Build history of the part. All positions in model axes, mm. Round coordinates to 2 decimals unless told otherwise and drop trailing zeros. Write each loop counter-clockwise with the first axis right and the second up, starting at its lowest first coordinate (ties: lowest second). Pieces come first, ordered by that corner, then holes.
1) Saw through at B-B (z = 101.6). Write the cut outline in (x, y) (3 decimals).
2) Flat gauge pins, fed straight in: pin 1 (6 mm diameter, centred on x = 28.02, z = 190.5, fed in from -Y); pin 2 (1 mm diameter, centred on x = 18, y = 14.5, fed in from -Z). Where does each tip first touch, or does it go through?
3) Wall check: probe 1 along X at (y, z) = (14.9, 97.5); probe 2 along X at (y, z) = (14.85, 190.5); probe 3 along X at (y, z) = (13.85, 180). Give the ranges that are in metal, low to high.
4) Pull direction Z, two halves, no side cores. Call faces 1 (the flat face through (39.48, 14.27, 54.83)), 2 (the flat face through (-1, 12.7, 114)), 3 (the cylindrical face through (-54.223, 14.31, 115.586)), 4 (the cylindrical face through (28.89, 14.31, 192.19)): +Z half, -Z half, draft (parallel to the pull), parting line (faces both ways), or undercut.
5) Saw through at C-C (y = 15.15). State how many separate pieces and enclosed holes the cut face has, plus the area to 3 significant figures.
6) Saw through at A-A (x = -24.5). Write the cut outline in (y, z) (3 decimals).
7) Saw through at D-D (z = -4). Write the cut outline in (x, y) (3 decimals), plus the area to 3 significant figures.
from build123d import *

# Parameters (mm, degrees)
SKETCH3_W                = 114.3
SKETCH3_H                = 88.9
SKETCH3_W_2              = 101.6
SKETCH3_H_2              = 76.2
BOSS_EXTRUDE1_DEPTH      = 12.7
BOSS_EXTRUDE1_DEPTH_BACK = 12.7
SKETCH4_W                = 114.3
SKETCH4_H                = 88.9
BOSS_EXTRUDE2_DEPTH      = 3.175
BOSS_EXTRUDE3_DEPTH      = 3.175
SKETCH7_W                = 44.45
SKETCH7_H                = 25.4
BOSS_EXTRUDE4_DEPTH      = 6.35
SKETCH6_R                = 9.9695
CUT_EXTRUDE1_DEPTH       = 115.3
SKETCH13_W               = 29.21
SKETCH13_H               = 25.4
BOSS_EXTRUDE5_DEPTH      = 4.064
SKETCH14_W               = 6.35
SKETCH14_H               = 2.54
CUT_EXTRUDE2_DEPTH       = 31.75
SKETCH18_W               = 10.16
SKETCH18_H               = 5.08
CUT_EXTRUDE3_DEPTH       = 6.35
SKETCH19_R               = 0.635
CUT_EXTRUDE4_DEPTH       = 25.4
SKETCH20_R               = 1.905
CUT_EXTRUDE7_DEPTH       = 3.175
SKETCH23_R               = 5.08
SKETCH23_R_2             = 1.905
SKETCH23_R_3             = 2.38125
CUT_EXTRUDE8_DEPTH       = 3.175
SKETCH24_R               = 1.25
CUT_EXTRUDE9_DEPTH       = 3.175
BOSS_EXTRUDE7_DEPTH      = 114.3
BOSS_EXTRUDE8_DEPTH      = 28.575
SKETCH25_R               = 15.875
SKETCH25_R_2             = 12.7
CUT_EXTRUDE10_DEPTH      = 32.75
FILLET1_R                = 9.525
FILLET2_R                = 5.08
FILLET3_R                = 9.525


with BuildPart() as part:
    # Sketch3 → Boss-Extrude1 (new body, two sides)
    with BuildSketch(Plane(origin=(0, 0, 0), x_dir=(1, 0, 0), z_dir=(0, 1, 0))) as boss_extrude1_sk:
        with Locations((0, -158.75)):
            Rectangle(SKETCH3_W, SKETCH3_H)
        with Locations((0, -158.75)):
            Rectangle(SKETCH3_W_2, SKETCH3_H_2, mode=Mode.SUBTRACT)
    extrude(amount=BOSS_EXTRUDE1_DEPTH)
    extrude(boss_extrude1_sk.sketch, amount=-BOSS_EXTRUDE1_DEPTH_BACK)

    # Sketch4 → Boss-Extrude2 (add)
    with BuildSketch(Plane.XZ.offset(12.7)):
        with Locations((0, 158.75)):
            Rectangle(SKETCH4_W, SKETCH4_H)
    extrude(amount=BOSS_EXTRUDE2_DEPTH)

    # Sketch7 → Boss-Extrude4 (add)
    with BuildSketch(Plane(origin=(0, -12.7, 0), x_dir=(1, 0, 0), z_dir=(0, 1, 0))):
        with Locations((-28.575, -133.35)):
            Rectangle(SKETCH7_W, SKETCH7_H)
        with Locations((28.575, -133.35)):
            Rectangle(SKETCH7_W, SKETCH7_H)
    extrude(amount=BOSS_EXTRUDE4_DEPTH)

    # Sketch6 → Cut-Extrude1 (cut, through all)
    with BuildSketch(Plane.ZY.offset(57.15)):
        with Locations((133.35, 0)):
            Circle(SKETCH6_R)
    extrude(amount=-CUT_EXTRUDE1_DEPTH, mode=Mode.SUBTRACT)

    # Sketch13 → Boss-Extrude5 (add)
    with BuildSketch(Plane(origin=(0, -12.7, 0), x_dir=(1, 0, 0), z_dir=(0, 1, 0))):
        with Locations((-20.955, -133.35)):
            Rectangle(SKETCH13_W, SKETCH13_H)
        with Locations((20.955, -133.35)):
            Rectangle(SKETCH13_W, SKETCH13_H)
    extrude(amount=BOSS_EXTRUDE5_DEPTH)

    # Sketch14 → Cut-Extrude2 (cut)
    with BuildSketch(Plane.XY.offset(146.05)):
        with Locations((-27.305, -10.414)):
            Rectangle(SKETCH14_W, SKETCH14_H)
        with Locations((-27.305, -3.81)):
            Rectangle(SKETCH14_W, SKETCH14_H)
        with Locations((27.305, -10.414)):
            Rectangle(SKETCH14_W, SKETCH14_H)
        with Locations((27.305, -3.81)):
            Rectangle(SKETCH14_W, SKETCH14_H)
    extrude(amount=-CUT_EXTRUDE2_DEPTH, mode=Mode.SUBTRACT)

    # Sketch18 → Cut-Extrude3 (cut)
    with BuildSketch(Plane.XY.offset(120.65)):
        with Locations((-43.18, 10.16)):
            Rectangle(SKETCH18_W, SKETCH18_H)
    extrude(amount=-CUT_EXTRUDE3_DEPTH, mode=Mode.SUBTRACT)

    # Sketch19 → Cut-Extrude4 (cut)
    with BuildSketch(Plane(origin=(0, 12.7, 0), x_dir=(1, 0, 0), z_dir=(0, 1, 0))):
        with Locations((-53.975, -117.475)):
            Circle(SKETCH19_R)
        with Locations((53.975, -117.475)):
            Circle(SKETCH19_R)
        with Locations((-53.975, -200.025)):
            Circle(SKETCH19_R)
        with Locations((53.975, -200.025)):
            Circle(SKETCH19_R)
    extrude(amount=-CUT_EXTRUDE4_DEPTH, mode=Mode.SUBTRACT)

    # Sketch26 → Boss-Extrude7 (add)
    with BuildSketch(Plane(origin=(57.15, 0, 0), x_dir=(0, 0, -1), z_dir=(1, 0, 0))):
        Polygon((-203.2, 12.7), (-203.454, 12.7), (-203.454, 15.875), (-204.724, 15.875), (-213.23138686, -15.875), (-203.2, -15.875), align=None)
    extrude(amount=-BOSS_EXTRUDE7_DEPTH)

    # Sketch27 → Boss-Extrude8 (add)
    with BuildSketch(Plane.XZ.offset(15.875)):
        Polygon((57.15, 171.45), (95.25, 171.45), (95.25, 128.27), (100.33, 128.27), (100.33, 176.536200973), (57.15, 184.15), align=None)
        Polygon((-100.33, 176.536200973), (-57.15, 184.15), (-57.15, 171.45), (-95.25, 171.45), (-95.25, 128.27), (-100.33, 128.27), align=None)
    extrude(amount=-BOSS_EXTRUDE8_DEPTH)

    # Fillet1
    fillet1_edges = [part.edges().sort_by_distance(p)[0] for p in [
        (57.15, -1.5875, 184.15),
        (100.33, -1.5875, 176.536200973),
        (95.25, -1.5875, 171.45),
        (-100.33, -1.5875, 176.536200973),
        (-57.15, -1.5875, 184.15),
        (-95.25, -1.5875, 171.45),
    ]]
    fillet(fillet1_edges, radius=FILLET1_R)

    # Fillet2
    fillet2_edges = [part.edges().sort_by_distance(p)[0] for p in [
        (57.15, -1.5875, 171.45),
        (-57.15, -1.5875, 171.45),
    ]]
    fillet(fillet2_edges, radius=FILLET2_R)

    # Fillet3
    fillet3_edges = [part.edges().sort_by_distance(p)[0] for p in [
        (97.79, -15.875, 128.27),
        (97.79, 12.7, 128.27),
        (-97.79, -15.875, 128.27),
        (-97.79, 12.7, 128.27),
    ]]
    fillet(fillet3_edges, radius=FILLET3_R)


with BuildPart() as body_2:
    # Sketch5 → Boss-Extrude3 (new body)
    with BuildSketch(Plane(origin=(0, 12.7, 0), x_dir=(1, 0, 0), z_dir=(0, 1, 0))):
        with BuildLine():
            Line((-21.304313257, 6.330628851), (-57.15, -114.3))
            Line((-57.15, -114.3), (-57.15, -203.2))
            Line((-57.15, -203.2), (57.15, -203.2))
            Line((57.15, -203.2), (57.15, -114.3))
            Line((57.15, -114.3), (21.304313257, 6.330628851))
            ThreePointArc((21.304313257, 6.330628851), (0, 22.225), (-21.304313257, 6.330628851))
        make_face()
    extrude(amount=BOSS_EXTRUDE3_DEPTH)

    # Sketch20 → Cut-Extrude7 (cut)
    with BuildSketch(Plane(origin=(0, 15.875, 0), x_dir=(1, 0, 0), z_dir=(0, 1, 0))):
        with Locations((-53.975, -117.475)):
            Circle(SKETCH20_R)
        with Locations((-53.975, -200.025)):
            Circle(SKETCH20_R)
        with Locations((53.975, -200.025)):
            Circle(SKETCH20_R)
        with Locations((53.975, -117.475)):
            Circle(SKETCH20_R)
    extrude(amount=-CUT_EXTRUDE7_DEPTH, mode=Mode.SUBTRACT)

    # Sketch23 → Cut-Extrude8 (cut)
    with BuildSketch(Plane(origin=(0, 15.875, 0), x_dir=(1, 0, 0), z_dir=(0, 1, 0))):
        with Locations((36.232509154, -183.804266718)):
            Circle(SKETCH23_R)
        with Locations((44.45, -177.108533435)):
            Circle(SKETCH23_R_2)
        with Locations((28.015018307, -190.5)):
            Circle(SKETCH23_R_2)
        with Locations((2.615018307, -174.727283435)):
            Circle(SKETCH23_R_3)
    extrude(amount=-CUT_EXTRUDE8_DEPTH, mode=Mode.SUBTRACT)

    # Sketch24 → Cut-Extrude9 (cut)
    with BuildSketch(Plane(origin=(0, 15.875, 0), x_dir=(1, 0, 0), z_dir=(0, 1, 0))):
        with Locations((0, 9.5)):
            Circle(SKETCH24_R)
        with Locations((0, -9.5)):
            Circle(SKETCH24_R)
        with Locations((-8, 0)):
            Circle(SKETCH24_R)
        with Locations((8, 0)):
            Circle(SKETCH24_R)
    extrude(amount=-CUT_EXTRUDE9_DEPTH, mode=Mode.SUBTRACT)

    # Sketch25 → Cut-Extrude10 (cut, through all)
    with BuildSketch(Plane(origin=(0, 15.875, 0), x_dir=(1, 0, 0), z_dir=(0, 1, 0))):
        with Locations((0, -38.1)):
            Circle(SKETCH25_R)
        with Locations((-25.4, -101.6)):
            Circle(SKETCH25_R_2)
        with Locations((25.4, -101.6)):
            Circle(SKETCH25_R_2)
    extrude(amount=-CUT_EXTRUDE10_DEPTH, mode=Mode.SUBTRACT)


solid = body_2.part
Evaluation:
1. outline: (-53.376, 12.7) - (-38.1, 12.7) - (-38.1, 15.875) - (-53.376, 15.875) - close; (-12.7, 12.7) - (12.7, 12.7) - (12.7, 15.875) - (-12.7, 15.875) - close; (38.1, 12.7) - (53.376, 12.7) - (53.376, 15.875) - (38.1, 15.875) - close
2. pin 1: stops at y = 12.7
2. pin 2: stops at z = -13.7
3. probe 1: x = -52.16 to -37.42, -13.38 to 13.38, 37.42 to 52.16
3. probe 2: x = -57.15 to 26.11, 29.92 to 57.15
3. probe 3: x = -57.15 to 32.87, 39.6 to 57.15
4. face 1: -Z half
4. face 2: draft
4. face 3: undercut
4. face 4: undercut
5. separate pieces: 1
5. enclosed holes: 15
5. area: 18,100 mm2
6. outline: (12.7, 4.424) - (15.875, 4.424) - (15.875, 88.932) - (12.7, 88.932) - close; (12.7, 114.268) - (15.875, 114.268) - (15.875, 203.2) - (12.7, 203.2) - close
7. outline: (-21.997, 12.7) - (21.997, 12.7) - (21.997, 15.875) - (-21.997, 15.875) - close
7. area: 140 mm2
